For this review, take the finished solid that the model builds, in its own axes (mm). A direction names the side the tool comes from. Give positions to 0.01 mm unless a question says otherwise; leave off trailing zeros. Write each loop counter-clockwise with the first axis right and the second up, starting at its lowest first coordinate (ties: lowest second). Pieces come first, ordered by that corner, then holes. Notation, with made-up numbers: (-27, 58.25) -> (-8, 58.25) arc R31 cw to (-8, 95.25) -> close; hole circle Ø5 at (79.25, 65). An arc over 180 degrees is marked (long way). Return JSON: item names as keys, results as strings.
from build123d import *

# Parameters (mm, degrees)
BOX001_W         = 65
BOX001_H         = 31
BOX001_DEPTH     = 8
FILLET001_R      = 5
THICKNESS001_T   = 1.5
SKETCH002_W      = 14
SKETCH002_H      = 2.5
POCKET001_DEPTH  = 1.5
SKETCH003_R      = 2.5
PAD001_DEPTH     = 9.3
HOLE_D           = 2.2
HOLE_CBORE_D     = 4
HOLE_CBORE_DEPTH = 2
SKETCH005_R      = 10
POCKET002_DEPTH  = 1.5
CHAMFER_SIZE     = 1.3


with BuildPart() as part:
    # Box001 → Box001 (join)
    with BuildSketch(Plane.XY.offset(8)):
        with Locations((32.5, 15.5)):
            Rectangle(BOX001_W, BOX001_H)
    extrude(amount=BOX001_DEPTH)

    # Fillet001
    fillet001_edges = [part.edges().sort_by_distance(p)[0] for p in [
        (65, 0, 12),
        (65, 31, 12),
        (0, 0, 12),
        (0, 31, 12),
    ]]
    fillet(fillet001_edges, radius=FILLET001_R)

    # Thickness001
    thickness001_openings = [part.faces().sort_by_distance(p)[0] for p in [
        (32.5, 15.5, 8),
    ]]
    offset(amount=THICKNESS001_T, openings=thickness001_openings, kind=Kind.INTERSECTION)

    # Sketch002 (on Face19 of Thickness001) → Pocket001 (cut)
    with BuildSketch(Plane.YZ.offset(66.5)):
        with Locations((15.25, 9.25)):
            Rectangle(SKETCH002_W, SKETCH002_H)
    extrude(amount=-POCKET001_DEPTH, mode=Mode.SUBTRACT)

    # Sketch003 (on Face2 of Pocket001) → Pad001 (join)
    with BuildSketch(Plane(origin=(0, 0, 16), x_dir=(1, 0, 0), z_dir=(0, 0, -1))):
        with Locations((59.085, -3.845)):
            Circle(SKETCH003_R)
        with Locations((59.085, -27.155)):
            Circle(SKETCH003_R)
        with Locations((5.915, -27.155)):
            Circle(SKETCH003_R)
        with Locations((5.915, -3.845)):
            Circle(SKETCH003_R)
    extrude(amount=PAD001_DEPTH)

    # Hole (through all)
    with Locations(Plane.XY.offset(17.5)):
        with Locations((5.915, 27.155), (59.085, 27.155), (59.085, 3.845), (5.915, 3.845)):
            CounterBoreHole(HOLE_D / 2, HOLE_CBORE_D / 2, HOLE_CBORE_DEPTH)

    # Sketch005 (on Face30 of Hole) → Pocket002 (cut)
    with BuildSketch(Plane.XY.offset(17.5)):
        with Locations((40, 15)):
            Circle(SKETCH005_R)
    extrude(amount=-POCKET002_DEPTH, mode=Mode.SUBTRACT)

    # Chamfer
    chamfer_edges = [part.edges().sort_by_distance(p)[0] for p in [
        (56.585, 3.845, 16),
        (56.585, 27.155, 16),
        (3.415, 3.845, 16),
        (3.415, 27.155, 16),
    ]]
    chamfer(chamfer_edges, length=CHAMFER_SIZE)


solid = part.part
1. For pin 1 (2.5 mm diameter, centred on x = 59.085, y = 27.155, fed in from +Z); pin 2 (1.6 mm diameter, centred on x = 66, z = 10, fed in from +Y); pin 3 (9.5 mm diameter, centred on x = 23.5, y = 9.5, fed in from -Z), all flat-tipped, find the tip position at first contact; note any pin that passes through.
Results found:
{"pin 1": "stops at z = 15.5", "pin 2": "stops at y = 29.9", "pin 3": "stops at z = 16"}
2. For faces 4 (the flat face through (7, 26, 15.5)), 5 (the flat face through (32, 31, 12)), 6 (the flat face through (66, 15, 10.5)), list the 3-axis set-ups (+Z, -Z, +X, -X, +Y, -Y) from which the entire face can be reached by the end or side of a thin tool; tool diameter is ignored.
Results found:
{"face 4": "+Z", "face 5": "-Z", "face 6": "-Z, +X"}
3. To check wall thickness, follow probe 1 along Y at (x, z) = (37.5, 9.75); probe 2 along X at (y, z) = (18, 15); probe 3 along Y at (x, z) = (39.5, 17.25). State the ranges of each line that lie inside material, in increasing order.
Results found:
{"probe 1": "y = -1.5 to 0, 31 to 32.5", "probe 2": "x = -1.5 to 0, 65 to 66.5", "probe 3": "y = -1.5 to 5.01, 24.99 to 32.5"}
4. Add section B-B, the plane y = 15. State the section outline as (x, z) points, plus the area to 4 significant figures.
Results found:
{"outline": "(-1.5, 8) -> (0, 8) -> (0, 16) -> (30, 16) -> (30, 17.5) -> (-1.5, 17.5) -> close; (50, 16) -> (65, 16) -> (65, 10.5) -> (66.5, 10.5) -> (66.5, 17.5) -> (50, 17.5) -> close", "area": "92.25 mm²"}
5. Add section C-C, the plane z = 14. Count the separate pieces of the cut face and the enclosed holes in it, plus the area to 3 significant figures.
Results found:
{"separate pieces": "5", "enclosed holes": "5", "area": "346 mm²"}
6. Add section D-D, the plane x = 27.5. State the section outline as (y, z) points.
Results found:
{"outline": "(-1.5, 8) -> (0, 8) -> (0, 16) -> (31, 16) -> (31, 8) -> (32.5, 8) -> (32.5, 17.5) -> (-1.5, 17.5) -> close"}
7. Add section A-A, the plane x = 40. State the section outline as (y, z) points.
Results found:
{"outline": "(-1.5, 8) -> (0, 8) -> (0, 16) -> (5, 16) -> (5, 17.5) -> (-1.5, 17.5) -> close; (25, 16) -> (31, 16) -> (31, 8) -> (32.5, 8) -> (32.5, 17.5) -> (25, 17.5) -> close"}
8. The part is to be moulded in two halves that separate along X. For faces 1 (the cylindrical face through (64.646, 30.545, 12.817)), 2 (the flat face through (-1.5, 15, 13)), 3 (the cylindrical face through (5.655, 29.138, 16.514)), say which applies: +X half, -X half, draft (parallel to the pull), parting line (faces both ways), or undercut.
Results found:
{"face 1": "+X half", "face 2": "-X half", "face 3": "undercut"}
